Autodesk Inventor part; units mm, degrees
ref_plane "YZ Plane" through (0, 0, 0) normal (1, 0, 0) x (0, 1, 0)
ref_plane "XZ Plane" through (0, 0, 0) normal (0, 1, 0) x (-1, 0, 0)
ref_plane "XY Plane" through (0, 0, 0) normal (0, 0, 1) x (1, 0, 0)
sketch "Sketch1" plane through (0, 0, 0) normal (0, 1, 0) x (-1, 0, 0)
  line L0 (0, 0) -> (20, 0)
  line L1 (20, 0) -> (20, -50)
  line L2 (20, -50) -> (0, -50)
  line L3 (0, -50) -> (0, 0)
  line L4 (0, -50) -> (48, -50)
  line L5 (48, -50) -> (48, -30)
  line L6 (48, -30) -> (0, -30)
  line L7 (0, -30) -> (0, -50)
  circle A0 centre (10, -10) radius 3
  circle A1 centre (10, -30) radius 3
  line L8 (20, -50) -> (20, -36)
  line L9 (20, -36) -> (31, -36)
  line L10 (31, -36) -> (36.25, -36)
  circle A2 centre (36.25, -36) radius 2
  line L11 (36.25, -36) -> (43.25, -36)
  circle A3 centre (43.25, -36) radius 2
  line L12 (39.75, -36) -> (39.75, -44)
  circle A4 centre (39.75, -44) radius 2
  point P0 (20, -30)
  dimension "d0" = 20
  dimension "d1" = 50
  dimension "d2" = 48
  dimension "d3" = 20
  dimension "d4" = 6
  dimension "d5" = 6
  dimension "d6" = 10
  dimension "d7" = 10
  dimension "d8" = 20
  dimension "d9" = 10
  dimension "d10" = 11
  dimension "d11" = 5.25
  dimension "d12" = 14
  dimension "d13" = 4
  dimension "d14" = 7
  dimension "d15" = 4
  dimension "d21" = 8
  dimension "d22" = 4
extrude "Extrusion1" add sketch "Sketch1" along normal blind 6 contours L0 L1 L6 A1 L3 | L6 A1 L1 L2 L3 | L6 L5 L4 L1
fillet "Fillet1" radius 4 6 edges at (-20, 3, 0) (0, 3, 0) (-20, 3, -30) (-48, 3, -30) (-48, 3, -50) (0, 3, -50)
sketch "Sketch2" plane through (0, 6, 0) normal (0, 1, 0) x (1, 0, 0)
  line L0 (0, 0) -> (-20, 0)
  line L1 (-20, 0) -> (-20, 50)
  line L2 (-20, 50) -> (0, 50)
  line L3 (0, 50) -> (0, 0)
  circle A0 centre (-10, 30) radius 3
  circle A1 centre (-10, 30) radius 3
  circle A2 centre (-10, 10) radius 3
  circle A3 centre (-10, 10) radius 3
  dimension "d23" = 20
  dimension "d24" = 50
extrude "Extrusion2" add sketch "Sketch2" along normal blind 14
fillet "Fillet2" radius 5 3 edges at (0, 13, -50) (0, 13, 0) (-20, 13, 0)
fillet "Fillet3" radius 5 1 edges at (-20, 13, -50)
properties part number "CableChain_Mount"
Geometry: final body of the model. Coordinates: model frame, mm. A direction names the side the tool comes from. Give positions to 0.01 mm unless a question says otherwise; leave off trailing zeros. Write each loop counter-clockwise with the first axis right and the second up, starting at its lowest first coordinate (ties: lowest second). Pieces come first, ordered by that corner, then holes. Notation, with made-up numbers: (2, 67.25) -> (49, 67.25) arc R20 cw to (49, 99.25) -> close; hole circle Ø7 at (13.5, -39). An arc over 180 degrees is marked (long way). Answer in a Markdown table with one row per item.
(1) Set-up query: faces 5 (the flat face through (-18, 0, -30)), 6 (the flat face through (-20, 12, -25)), 7 (the cylindrical face through (-18, 13, -49)). Return all of +Z, -Z, +X, -X, +Y, -Y with unobstructed straight access to the full face (end or side cutting, diameter ignored); none if empty.
Answers below:
| item | result |
|---|---|
| face 5 | +Z, -Z, +X, -X, -Y |
| face 6 | +Z, -X, +Y |
| face 7 | -Z, -X, +Y |
(2) Section query B-B on y = 15.5. Return loops of the section in (x, z), then the cut area to 3 significant figures.
Answers below:
| item | result |
|---|---|
| outline | (-20, -45) arc R5 ccw to (-15, -50) -> (-5, -50) arc R5 ccw to (0, -45) -> (0, -5) arc R5 ccw to (-5, 0) -> (-15, 0) arc R5 ccw to (-20, -5) -> close; hole circle Ø6 at (-10, -30); hole circle Ø6 at (-10, -10) |
| area | 922 mm^2 |
(3) Draft query along X for faces 1 (the flat face through (-34, 3, -30)), 2 (the cylindrical face through (-19, 10, -2)), 3 (the cylindrical face through (-37.173, 2.958, -34.226)), 4 (the cylindrical face through (-39.316, 2.958, -42.048)). Return one class per face: +X half, -X half, draft (parallel to the pull), parting line (faces both ways), or undercut.
Answers below:
| item | result |
|---|---|
| face 1 | draft |
| face 2 | -X half |
| face 3 | undercut |
| face 4 | undercut |
(4) Section query D-D on x = -36.25. Return loops of the section in (y, z).
Answers below:
| item | result |
|---|---|
| outline | (0, -50) -> (6, -50) -> (6, -38) -> (0, -38) -> close; (0, -34) -> (6, -34) -> (6, -30) -> (0, -30) -> close |
(5) Section query C-C on z = -36. Return loops of the section in (x, y), then the cut area to 3 significant figures.
Answers below:
| item | result |
|---|---|
| outline | (-48, 0) -> (-45.25, 0) -> (-45.25, 6) -> (-48, 6) -> close; (-41.25, 0) -> (-38.25, 0) -> (-38.25, 6) -> (-41.25, 6) -> close; (-34.25, 0) -> (0, 0) -> (0, 20) -> (-20, 20) -> (-20, 6) -> (-34.25, 6) -> close |
| area | 520 mm^2 |
(6) Pin query (flat end, axial travel): pin 1 (12 mm diameter, centred on y = 15.5, z = -44.5, fed in from -X); pin 2 (10 mm diameter, centred on x = -30.5, z = -28, fed in from +Y); pin 3 (3 mm diameter, centred on x = -29, y = 3.5, fed in from +Z). Return the tip coordinate at first contact, or that it passes through.
Answers below:
| item | result |
|---|---|
| pin 1 | x = -20 |
| pin 2 | y = 6 |
| pin 3 | z = -30 |
(7) Section query A-A on z = -10. Return loops of the section in (x, y), then the cut area to 3 significant figures.
Answers below:
| item | result |
|---|---|
| outline | (-20, 0) -> (-13, 0) -> (-13, 20) -> (-20, 20) -> close; (-7, 0) -> (0, 0) -> (0, 20) -> (-7, 20) -> close |
| area | 280 mm^2 |
(8) Ray query, line 1 along X through (y, z) = (2.15, -36); line 2 along Z through (x, y) = (-10, 4.6); line 3 along X through (y, z) = (2.95, -44). Return the intervals inside material, ascending. Write a range as [from, to].
Answers below:
| item | result |
|---|---|
| line 1 | [-48, -45.25], [-41.25, -38.25], [-34.25, 0] |
| line 2 | [-50, -33], [-27, -13], [-7, 0] |
| line 3 | [-48, -41.75], [-37.75, 0] |
